Input: dimensioned drawing with shaded views. Units: mm. Origin: part minimum x, y, z. A direction names the side the tool comes from. Round coordinates to 2 decimals unless told otherwise and drop trailing zeros. Loops run counter-clockwise (first coordinate to the right, second up) from the corner with the lowest first, then second, coordinate; pieces in that order, holes last. Notation, with made-up numbers: (36.5, 15.5) - (92.5, 15.5) arc R29 cw to (92.5, 38.5) - close; hole circle Ø11 at (-31, 33.25). An arc over 180 degrees is marked (long way). One line per question, with ' | ' between items. Start each with the question number.
1. Cut plane C-C (z = 14.75). Return loops of the section in (x, y).
2. Cut plane B-B (x = 14). Return loops of the section in (y, z), then the cut area to 3 significant figures.
3. Cut plane D-D (x = 2). Return loops of the section in (y, z).
4. Mould query, pull axis Z, two halves, no side actions, for the marked faces 1, 2, 3 and 4. Classes: pulls with the +Z half, pulls with the -Z half, needs draft (parallel to the pull), parting line crosses it, or undercut.
5. Access query for the marked faces 5 and 6. Directions: +Z, -Z, +X, -X, +Y, -Y. A direction counts if a zero-diameter tool reaches every point of the face in a straight line with its end or side. Return the directions, or none.
6. Ray query, line 1 (Y direction, x = 4.5, z = 5); line 2 (X direction, y = 8.5, z = 8.25); line 3 (Z direction, x = 13, y = 12.75). Return the intervals inside material, ascending.
7. Pin query (flat end, axial travel): pin 1 (3 mm diameter, centred on x = 11.5, z = 5.5, fed in from -Y); pin 2 (6 mm diameter, centred on x = 4, y = 7.5, fed in from -Z); pin 3 (1.5 mm diameter, centred on y = 3, z = 5.5, fed in from -X). Return the tip coordinate at first contact, or that it passes through.
8. Cut plane A-A (y = 12). Return loops of the section in (x, z), then the cut area to 3 significant figures.
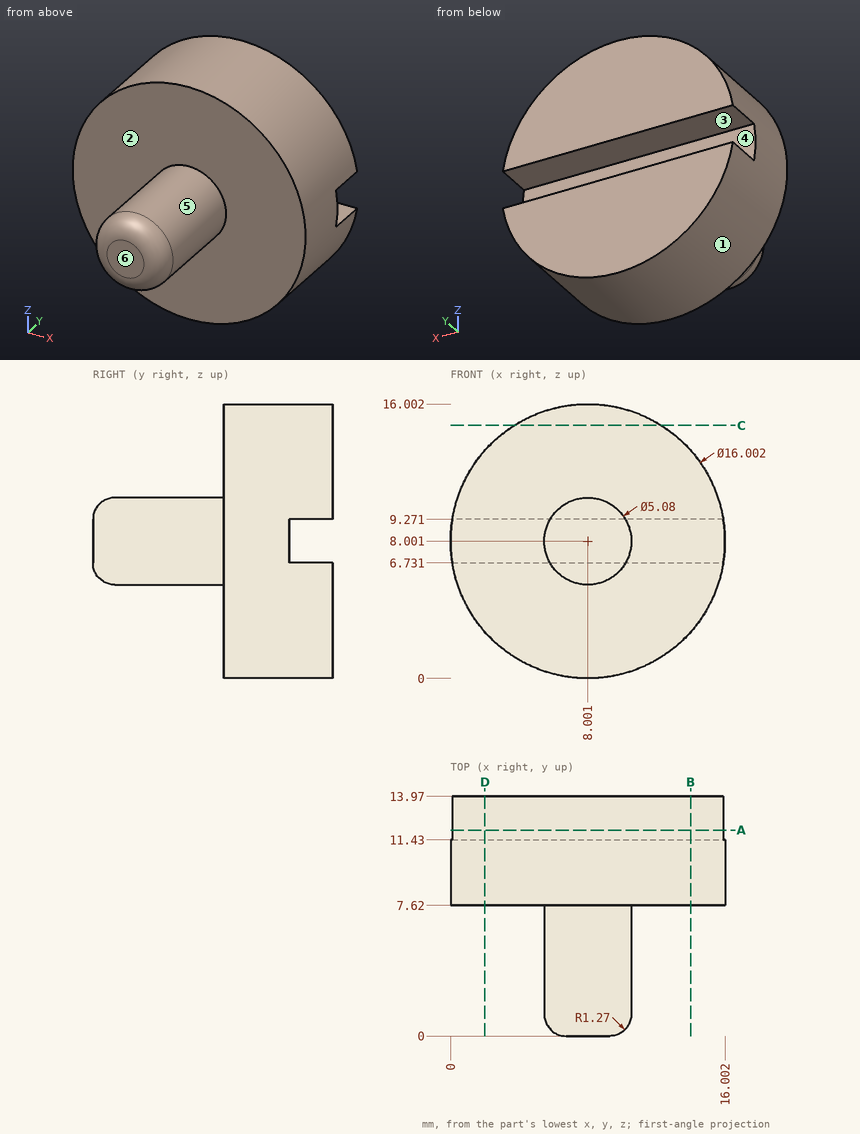
Answers follow:
1) outline: (3.7, 7.62) - (12.3, 7.62) - (12.3, 13.97) - (3.7, 13.97) - close
2) outline: (7.62, 2.71) - (13.97, 2.71) - (13.97, 6.73) - (11.43, 6.73) - (11.43, 9.27) - (13.97, 9.27) - (13.97, 13.3) - (7.62, 13.3) - close | area: 60.8 mm2
3) outline: (7.62, 2.71) - (13.97, 2.71) - (13.97, 6.73) - (11.43, 6.73) - (11.43, 9.27) - (13.97, 9.27) - (13.97, 13.29) - (7.62, 13.29) - close
4) face 1: parting line crosses it | face 2: needs draft | face 3: undercut | face 4: undercut
5) face 5: -Y | face 6: +Z, -Z, +X, -X, -Y
6) line 1: y = 7.62 to 13.97 | line 2: x = 0 to 16 | line 3: z = 1.75 to 6.73, 9.27 to 14.25
7) pin 1: stops at y = 7.62 | pin 2: stops at z = 0.06 | pin 3: stops at x = 6.16
8) outline: (0.1, 6.73) arc R8 ccw to (15.9, 6.73) - close; (0.1, 9.27) - (15.9, 9.27) arc R8 ccw to start | area: 161 mm2
